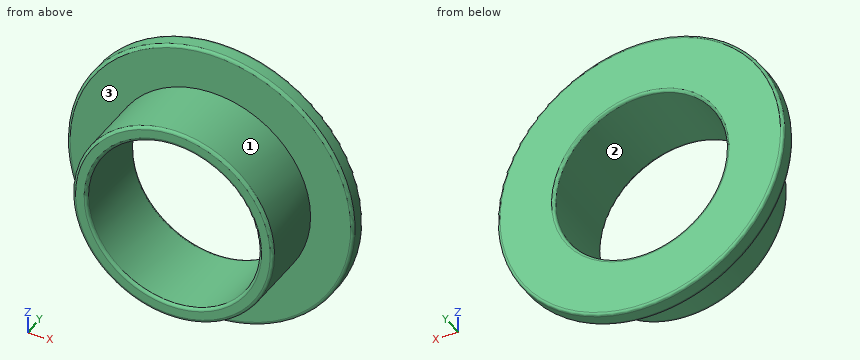
from build123d import *

# Parameters (mm, degrees)
SKETCH1_R           = 7
SKETCH1_R_2         = 6
BOSS_EXTRUDE1_DEPTH = 6
BOSS_EXTRUDE2_START = -1.2
SKETCH2_R           = 10
SKETCH2_R_2         = 6
BOSS_EXTRUDE2_DEPTH = 1.2
FILLET1_R           = 0.2


with BuildPart() as part:
    # Sketch1 → Boss-Extrude1 (new body)
    with BuildSketch(Plane(origin=(0, 0, 0), x_dir=(1, 0, 0), z_dir=(0, 1, 0))):
        with Locations(Location((0, 0, 0), (0, 0, 270))):
            Circle(SKETCH1_R)
        with Locations(Location((0, 0, 0), (0, 0, 270))):
            Circle(SKETCH1_R_2, mode=Mode.SUBTRACT)
    extrude(amount=BOSS_EXTRUDE1_DEPTH)

    # Sketch2 → Boss-Extrude2 (add)
    with BuildSketch(Plane(origin=(0, 6, 0), x_dir=(1, 0, 0), z_dir=(0, 1, 0)).offset(BOSS_EXTRUDE2_START)):
        with Locations(Location((0, 0, 0), (0, 0, 270))):
            Circle(SKETCH2_R)
        with Locations(Location((0, 0, 0), (0, 0, 270))):
            Circle(SKETCH2_R_2, mode=Mode.SUBTRACT)
    extrude(amount=BOSS_EXTRUDE2_DEPTH)

    # Fillet1
    fillet1_edges = [part.edges().sort_by_distance(p)[0] for p in [
        (0, 6, -10),
        (0, 4.8, -10),
        (0, 0, -7),
        (0, 0, -6),
        (0, 6, -6),
    ]]
    fillet(fillet1_edges, radius=FILLET1_R)


solid = part.part
Could you check a few things on this model? Use its own coordinates, in mm. Face numbers are marked on the shaded views. Give positions to 0.01 mm unless a question says otherwise; leave off trailing zeros. Order: outer loops, then holes, each group sorted by start corner. A loop starts at its lowest first (then second) coordinate and runs counter-clockwise, first axis right, second up.
1. Suppose I cut it at C-C (y = 2.1). List the corners of the cut face in (x, z) for me.
2. Suppose I cut it at A-A (x = 0). List the corners of the cut face in (y, z) for me.
3. Suppose I cut it at D-D (y = 5.55). List the corners of the cut face in (x, z) for me.
4. We'd pull the mould along X, two halves only. Please class the marked faces 1, 2 and 3: pulls with the +X half, pulls with the -X half, needs draft (parallel to the pull), parting line crosses it, or undercut.
5. Will these pins go through, and if not, where does the flat tip stop? P1, Ø1, axis at y = 4.5, z = -2, coming from the -X side; P2, Ø1, axis at x = 3.5, y = 3, coming from the +Z side; P3, Ø2, axis at y = 0.5, z = 1.5, coming from the +X side.
6. Suppose I cut it at B-B (z = 0). List the corners of the cut face in (x, y) for me, plus the area to 3 significant figures.
7. I need wall thicknesses on L1, parallel to X at y = 2.9, z = 0; L2, parallel to Y at x = -6.75, z = 4.5; L3, parallel to X at y = 1.05, z = 3.25. Which ranges of each line are inside material? Lowest first, please.
Solved:
1. outline: circle Ø14 at (0, 0); hole circle Ø12 at (0, 0)
2. outline: (0, -6.8) arc R0.2 ccw to (0.2, -7) - (4.8, -7) - (4.8, -9.8) arc R0.2 ccw to (5, -10) - (5.8, -10) arc R0.2 ccw to (6, -9.8) - (6, -6.2) arc R0.2 ccw to (5.8, -6) - (0.2, -6) arc R0.2 ccw to (0, -6.2) - close; (0, 6.2) arc R0.2 ccw to (0.2, 6) - (5.8, 6) arc R0.2 ccw to (6, 6.2) - (6, 9.8) arc R0.2 ccw to (5.8, 10) - (5, 10) arc R0.2 ccw to (4.8, 9.8) - (4.8, 7) - (0.2, 7) arc R0.2 ccw to (0, 6.8) - close
3. outline: circle Ø20 at (0, 0); hole circle Ø12 at (0, 0)
4. face 1: parting line crosses it
4. face 2: undercut
4. face 3: needs draft
5. P1: stops at x = -9.83
5. P2: stops at z = 6.32
5. P3: stops at x = 6.98
6. outline: (-10, 5) arc R0.2 ccw to (-9.8, 4.8) - (-7, 4.8) - (-7, 0.2) arc R0.2 ccw to (-6.8, 0) - (-6.2, 0) arc R0.2 ccw to (-6, 0.2) - (-6, 5.8) arc R0.2 ccw to (-6.2, 6) - (-9.8, 6) arc R0.2 ccw to (-10, 5.8) - close; (6, 0.2) arc R0.2 ccw to (6.2, 0) - (6.8, 0) arc R0.2 ccw to (7, 0.2) - (7, 4.8) - (9.8, 4.8) arc R0.2 ccw to (10, 5) - (10, 5.8) arc R0.2 ccw to (9.8, 6) - (6.2, 6) arc R0.2 ccw to (6, 5.8) - close
6. area: 19.1 mm2
7. L1: x = -7 to -6, 6 to 7
7. L2: y = 4.8 to 6
7. L3: x = -6.2 to -5.04, 5.04 to 6.2
